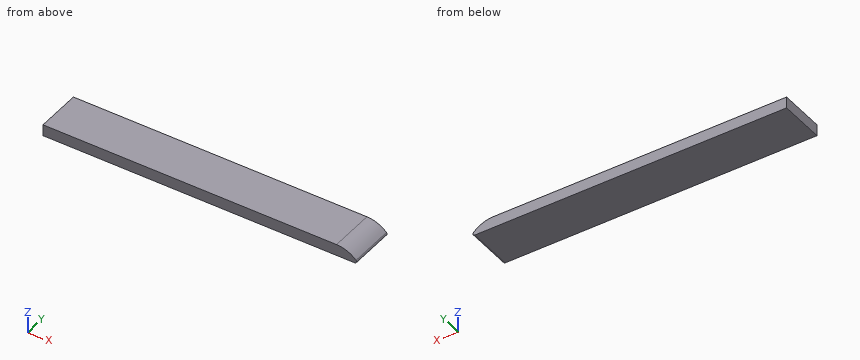
```python
from build123d import *

# Parameters (mm, degrees)
F0_W        = 704.85
F0_H        = 101.6
F1_DEPTH    = 25.4
F2_T1_DEPTH = 350.0928592435
F3_R        = 4.2426380505


# Not quite as in the source:
# - a fillet or chamfer that OpenCascade refuses, or shapes differently, is made with other operations: its cross-section is extruded or revolved along the edge and cut away or added


with BuildPart() as f1:
    # F0 (on Top) → F1 (new body)
    with BuildSketch(Plane.XY):
        with Locations((25.5663767457, 11.9668386396)):
            Rectangle(F0_W, F0_H)
    extrude(amount=F1_DEPTH)

    # F2: fillet of radius 61.3210244843 on 1 edges, made by hand

    # F2_s2 → F2_t1 (cut)
    with BuildSketch(Plane.XZ.offset(-187.0132682614)):
        with BuildLine():
            ThreePointArc((377.9913767457, 0), (356.1993813791, 18.6820068679), (328.292804897, 25.4))
            Line((328.292804897, 25.4), (377.9913767457, 25.4))
            Line((377.9913767457, 25.4), (377.9913767457, 0))
        make_face()
    extrude(amount=F2_T1_DEPTH, mode=Mode.SUBTRACT)

    # F3
    f3_edges = [f1.edges().sort_by_distance(p)[0] for p in [
        (377.991377, 11.966839, 0),
    ]]
    fillet(f3_edges, radius=F3_R)


solid = f1.part
```
Design review of the part built by this model. Coordinates are the model's own, in mm. Coordinates: 2 decimals unless noted, no trailing zeros. Loops run counter-clockwise (first coordinate to the right, second up) from the corner with the lowest first, then second, coordinate; pieces in that order, holes last. Notation, with made-up numbers: (6.25, 4) - (26.25, 4) arc R25 cw to (26.25, 21) - close; hole circle Ø11 at (73.25, 55). An arc over 180 degrees is marked (long way). Use CSV: the item, a comma, the result in double quotes. Start each with the question number.
1) Consider section A-A on y = 6. Write out the cut boundary in (x, z).
2) Consider section B-B on z = 19.5. Write out the cut boundary in (x, y).
3) Wall thickness on L1, parallel to X at y = -1, z = 4.75; L2, parallel to X at y = 0, z = 19.75: over which ranges is each line inside the solid? List them lowest first. Write a range as from..to.
4) For pin 1 Ø5 at (y, z) = (-7.5, 18.5) entering from +X, flat-tipped, find the tip position at first contact; note if it passes through.
Geometry says:
1,outline,"(-326.86, 0) - (368.85, 0) arc R4.24 ccw to (371.86, 7.23) arc R61.32 ccw to (328.29, 25.4) - (-326.86, 25.4) - close"
2,outline,"(-326.86, -38.83) - (354.54, -38.83) - (354.54, 62.77) - (-326.86, 62.77) - close"
3,L1,"-326.86..373.06"
3,L2,"-326.86..354"
4,pin 1,"x = 360.92"
